from build123d import *

# Parameters (mm, degrees)
F1_DEPTH = 25
F3_COUNT = 20
F3_ANGLE = 342
F5_R     = 12.5
F6_DEPTH = 53.5


with BuildPart() as f1:
    # F0 (on Front) → F1 (new body)
    with BuildSketch(Plane.XZ):
        with BuildLine():
            ThreePointArc((-2.524062, 17.317018), (-11.447247, -13.236712), (17.5, 0))
            ThreePointArc((17.5, 0), (13.236712, 11.447247), (2.524062, 17.317018))
            ThreePointArc((2.524062, 17.317018), (0, 17.5), (-2.524062, 17.317018))
        make_face()
        with BuildLine():
            ThreePointArc((-2.524062, 17.317018), (0, 17.5), (2.524062, 17.317018))
            Line((2.524062, 17.317018), (1.57, 19.938282))
            Line((1.57, 19.938282), (0.825231, 21.984517))
            ThreePointArc((0.825231, 21.984517), (0, 22), (-0.825231, 21.984517))
            Line((-0.825231, 21.984517), (-2.524062, 17.317018))
        make_face()
    extrude(amount=F1_DEPTH)


with BuildPart() as f3_1:
    # F3: instance of F1
    add(f1.part.rotate(Axis((0, -51.437987, 0), (0, 1, 0)), 1 * F3_ANGLE / (F3_COUNT - 1)))


with BuildPart() as f3_2:
    # F3: instance of F1
    add(f1.part.rotate(Axis((0, -51.437987, 0), (0, 1, 0)), 2 * F3_ANGLE / (F3_COUNT - 1)))


with BuildPart() as f3_3:
    # F3: instance of F1
    add(f1.part.rotate(Axis((0, -51.437987, 0), (0, 1, 0)), 3 * F3_ANGLE / (F3_COUNT - 1)))


with BuildPart() as f3_4:
    # F3: instance of F1
    add(f1.part.rotate(Axis((0, -51.437987, 0), (0, 1, 0)), 4 * F3_ANGLE / (F3_COUNT - 1)))


with BuildPart() as f3_5:
    # F3: instance of F1
    add(f1.part.rotate(Axis((0, -51.437987, 0), (0, 1, 0)), 5 * F3_ANGLE / (F3_COUNT - 1)))


with BuildPart() as f3_6:
    # F3: instance of F1
    add(f1.part.rotate(Axis((0, -51.437987, 0), (0, 1, 0)), 6 * F3_ANGLE / (F3_COUNT - 1)))


with BuildPart() as f3_7:
    # F3: instance of F1
    add(f1.part.rotate(Axis((0, -51.437987, 0), (0, 1, 0)), 7 * F3_ANGLE / (F3_COUNT - 1)))


with BuildPart() as f3_8:
    # F3: instance of F1
    add(f1.part.rotate(Axis((0, -51.437987, 0), (0, 1, 0)), 8 * F3_ANGLE / (F3_COUNT - 1)))


with BuildPart() as f3_9:
    # F3: instance of F1
    add(f1.part.rotate(Axis((0, -51.437987, 0), (0, 1, 0)), 9 * F3_ANGLE / (F3_COUNT - 1)))


with BuildPart() as f3_10:
    # F3: instance of F1
    add(f1.part.rotate(Axis((0, -51.437987, 0), (0, 1, 0)), 10 * F3_ANGLE / (F3_COUNT - 1)))


with BuildPart() as f3_11:
    # F3: instance of F1
    add(f1.part.rotate(Axis((0, -51.437987, 0), (0, 1, 0)), 11 * F3_ANGLE / (F3_COUNT - 1)))


with BuildPart() as f3_12:
    # F3: instance of F1
    add(f1.part.rotate(Axis((0, -51.437987, 0), (0, 1, 0)), 12 * F3_ANGLE / (F3_COUNT - 1)))


with BuildPart() as f3_13:
    # F3: instance of F1
    add(f1.part.rotate(Axis((0, -51.437987, 0), (0, 1, 0)), 13 * F3_ANGLE / (F3_COUNT - 1)))


with BuildPart() as f3_14:
    # F3: instance of F1
    add(f1.part.rotate(Axis((0, -51.437987, 0), (0, 1, 0)), 14 * F3_ANGLE / (F3_COUNT - 1)))


with BuildPart() as f3_15:
    # F3: instance of F1
    add(f1.part.rotate(Axis((0, -51.437987, 0), (0, 1, 0)), 15 * F3_ANGLE / (F3_COUNT - 1)))


with BuildPart() as f3_16:
    # F3: instance of F1
    add(f1.part.rotate(Axis((0, -51.437987, 0), (0, 1, 0)), 16 * F3_ANGLE / (F3_COUNT - 1)))


with BuildPart() as f3_17:
    # F3: instance of F1
    add(f1.part.rotate(Axis((0, -51.437987, 0), (0, 1, 0)), 17 * F3_ANGLE / (F3_COUNT - 1)))


with BuildPart() as f3_18:
    # F3: instance of F1
    add(f1.part.rotate(Axis((0, -51.437987, 0), (0, 1, 0)), 18 * F3_ANGLE / (F3_COUNT - 1)))


with BuildPart() as f3_19:
    # F3: instance of F1
    add(f1.part.rotate(Axis((0, -51.437987, 0), (0, 1, 0)), 19 * F3_ANGLE / (F3_COUNT - 1)))


with BuildPart() as f1_1:
    add(f1.part)

    # F4: union F3_19, F3_3, F3_11, F3_14, F3_5, F3_4, F3_8, F3_6, F3_7, F3_9, F3_10, F3_12, F3_15, F3_18, F3_13, F3_2, F3_16, F3_17, F3_1
    add(f3_19.part)
    add(f3_3.part)
    add(f3_11.part)
    add(f3_14.part)
    add(f3_5.part)
    add(f3_4.part)
    add(f3_8.part)
    add(f3_6.part)
    add(f3_7.part)
    add(f3_9.part)
    add(f3_10.part)
    add(f3_12.part)
    add(f3_15.part)
    add(f3_18.part)
    add(f3_13.part)
    add(f3_2.part)
    add(f3_16.part)
    add(f3_17.part)
    add(f3_1.part)

    # F5 (on face) → F6 (cut)
    with BuildSketch(Plane.XZ.offset(25)):
        Circle(F5_R)
    extrude(amount=-F6_DEPTH, mode=Mode.SUBTRACT)


solid = f1_1.part
The listing builds one solid part. Answer for the finished solid, in the listing's coordinates (mm). A direction names the side the tool comes from. Coordinates: 2 decimals unless noted, no trailing zeros. Loops run counter-clockwise (first coordinate to the right, second up) from the corner with the lowest first, then second, coordinate; pieces in that order, holes last. Notation, with made-up numbers: (58.5, 18.5) -> (115.5, 18.5) arc R21 cw to (115.5, 55.5) -> close; hole circle Ø2 at (15.5, 66). An arc over 180 degrees is marked (long way). Answer in a Markdown table with one row per item. Add a question column.
1. The part is cut by section B-B, the plane x = 0. Write down the section's boundary in (y, z), then the cut area to 3 significant figures.
2. Determine the mould class of faces 5 (the cylindrical face through (-17.79, -12.32, 12.94)), 6 (the flat face through (9, 0, -9)), 7 (the flat face through (14.9, -12.3, 12.9)), 8 (the cylindrical face through (6.787, -12.325, -20.927)) for opening direction Z: +Z half, -Z half, draft (parallel to the pull), parting line (faces both ways), or undercut.
3. For faces 1 (the cylindrical face through (20.92, -12.32, -6.81)), 2 (the flat face through (19.23, -12.32, -4.5)), 3 (the flat face through (-19.683, -12.325, -1.663)), 4 (the flat face through (-10.22, -12.32, -16.9)), determine the directions among +Z, -Z, +X, -X, +Y, -Y from which every point of the face is accessible in a straight line to the end or side of a thin tool.
4. The part is cut by section A-A, the plane z = 0. Write down the section's boundary in (x, y).
5. Consider line 1 (Z direction, x = 0, y = -21); line 2 (Z direction, x = -20, y = -21.25); line 3 (X direction, y = -8.75, z = 3). Determine where each line is inside the solid, lowest interval first. Write a range as [from, to].
6. Flat-ended cylindrical pins translate along their axes: P1, Ø2, axis at y = -8, z = -9.5, coming from the -X side; P2, Ø5, axis at y = -4, z = 13.5, coming from the +X side; P3, Ø1, axis at y = -6.5, z = -10.5, coming from the -X side; P4, Ø22.5, axis at x = 0, z = 0, coming from the -Y side. Find the tip coordinate at first contact, or state that the pin passes through.
Answer below:
| question | item | result |
|---|---|---|
| 1 | outline | (-25, -22) -> (0, -22) -> (0, -12.5) -> (-25, -12.5) -> close; (-25, 12.5) -> (0, 12.5) -> (0, 22) -> (-25, 22) -> close |
| 1 | area | 475 mm2 |
| 2 | face 5 | +Z half |
| 2 | face 6 | draft |
| 2 | face 7 | undercut |
| 2 | face 8 | -Z half |
| 3 | face 1 | -Z, +X, +Y, -Y |
| 3 | face 2 | +X, +Y, -Y |
| 3 | face 3 | -X, +Y, -Y |
| 3 | face 4 | -Z, +Y, -Y |
| 4 | outline | (-22, -25) -> (-12.5, -25) -> (-12.5, 0) -> (-22, 0) -> close; (12.5, -25) -> (22, -25) -> (22, 0) -> (12.5, 0) -> close |
| 5 | line 1 | [-22, -12.5], [12.5, 22] |
| 5 | line 2 | [-7.6, -5.1], [-1.55, 1.55], [5.1, 7.6] |
| 5 | line 3 | [-17.31, -12.13], [12.13, 17.31] |
| 6 | P1 | x = -17.09 |
| 6 | P2 | x = 18.27 |
| 6 | P3 | x = -17.42 |
| 6 | P4 | through |
